Can you work these out from the model? Positions are in its coordinate system, mm. A direction names the side the tool comes from. Round coordinates to 2 decimals unless told otherwise and drop trailing zeros. Loops run counter-clockwise (first coordinate to the right, second up) from the corner with the lowest first, then second, coordinate; pieces in that order, holes last. Notation, with made-up numbers: (57.5, -27.75) -> (73.5, -27.75) arc R22 ccw to (73.5, -9.75) -> close; hole circle Ø8 at (71.5, 10.25). An arc over 180 degrees is marked (long way). Write item = value, one per line.
from build123d import *

# Parameters (mm, degrees)
SKETCH1_W           = 150
SKETCH1_H           = 30
BOSS_EXTRUDE1_DEPTH = 5
SKETCH3_W           = 4
SKETCH3_H           = 30
BOSS_EXTRUDE2_DEPTH = 10
SKETCH4_W           = 4
SKETCH4_H           = 30
BOSS_EXTRUDE3_DEPTH = 10
FILLET1_R           = 2


with BuildPart() as part:
    # Sketch1 → Boss-Extrude1 (new body)
    with BuildSketch(Plane(origin=(0, 0, 0), x_dir=(1, 0, 0), z_dir=(0, 1, 0))):
        with Locations((75, 15)):
            Rectangle(SKETCH1_W, SKETCH1_H)
    extrude(amount=BOSS_EXTRUDE1_DEPTH)

    # Sketch3 → Boss-Extrude2 (add)
    with BuildSketch(Plane(origin=(0, 5, 0), x_dir=(1, 0, 0), z_dir=(0, 1, 0))):
        with Locations((148, 15)):
            Rectangle(SKETCH3_W, SKETCH3_H)
    extrude(amount=BOSS_EXTRUDE2_DEPTH)

    # Sketch4 → Boss-Extrude3 (add)
    with BuildSketch(Plane(origin=(0, 5, 0), x_dir=(1, 0, 0), z_dir=(0, 1, 0))):
        with Locations((2, 15)):
            Rectangle(SKETCH4_W, SKETCH4_H)
    extrude(amount=BOSS_EXTRUDE3_DEPTH)

    # Fillet1
    fillet1_edges = [part.edges().sort_by_distance(p)[0] for p in [
        (146, 15, -15),
        (4, 15, -15),
    ]]
    fillet(fillet1_edges, radius=FILLET1_R)


solid = part.part
1. Suppose I cut it at C-C, the plane x = 28. List the corners of the cut face in (y, z) for me.
Entries:
outline = (0, -30) -> (5, -30) -> (5, 0) -> (0, 0) -> close
2. We'd pull the mould along X, two halves only. Please class faces 3 (the flat face through (150, 7, -15)), 4 (the flat face through (4, 9, -15)), 5 (the flat face through (146, 9, -15)), 6 (the flat face through (75, 4, 0)): released by +X, released by -X, zero draft, split by the parting line, or undercut.
Entries:
face_3 = released by +X
face_4 = undercut
face_5 = undercut
face_6 = zero draft
3. I'm going to push a flat-ended pin straight in: pin 1 (9 mm diameter, centred on x = 97.5, z = -12.5, fed in from +Y). Where does the tip first touch, or does it pass through?
Entries:
pin_1 = 5
4. For faces 1 (the flat face through (74, 0, -15)), 2 (the flat face through (74, 5, -15)), which set-ups out of +Z, -Z, +X, -X, +Y, -Y let a thin tool reach every point of the face, with its end or its side?
Entries:
face_1 = +Z, -Z, +X, -X, -Y
face_2 = +Z, -Z, +Y
5. I need wall thicknesses on line 1 (X direction, y = 5.5, z = -3.75); line 2 (Y direction, x = 143.5, z = -9); line 3 (X direction, y = 13.75, z = -25.75). Which ranges of each line are inside material? Lowest first, please. Write a range as [from, to].
Entries:
line_1 = [0, 4], [146, 150]
line_2 = [0, 5]
line_3 = [0, 3.85], [146.15, 150]
6. Suppose I cut it at B-B, the plane z = -11.75. List the corners of the cut face in (x, y) for me.
Entries:
outline = (0, 0) -> (150, 0) -> (150, 15) -> (148, 15) arc R2 ccw to (146, 13) -> (146, 5) -> (4, 5) -> (4, 13) arc R2 ccw to (2, 15) -> (0, 15) -> close
7. Suppose I cut it at A-A, the plane y = 7.75. List the corners of the cut face in (x, z) for me, and give its area (3 significant figures).
Entries:
outline = (0, -30) -> (4, -30) -> (4, 0) -> (0, 0) -> close; (146, -30) -> (150, -30) -> (150, 0) -> (146, 0) -> close
area = 240 mm²
